```python
from build123d import *

# Parameters (mm, degrees)
SKETCH1_R           = 16.5
BOSS_EXTRUDE1_DEPTH = 6.5
BOSS_EXTRUDE1_TAPER = 6
SKETCH2_R           = 14.25
CUT_EXTRUDE1_DEPTH  = 4.5
CUT_EXTRUDE2_START  = -6
CUT_EXTRUDE2_DEPTH  = 6
CHAMFER1_SIZE       = 1.5


with BuildPart() as part:
    # Sketch1 → Boss-Extrude1 (new body)
    with BuildSketch(Plane(origin=(0, 0, 0), x_dir=(1, 0, 0), z_dir=(0, 1, 0))):
        Circle(SKETCH1_R)
    extrude(amount=BOSS_EXTRUDE1_DEPTH, taper=BOSS_EXTRUDE1_TAPER)

    # Sketch2 → Cut-Extrude1 (cut)
    with BuildSketch(Plane.XZ):
        with Locations(Location((0, 0, 0), (0, 0, 270))):
            Circle(SKETCH2_R)
    extrude(amount=-CUT_EXTRUDE1_DEPTH, mode=Mode.SUBTRACT)

    # Sketch3 → Cut-Extrude2 (cut)
    with BuildSketch(Plane(origin=(0, 6.5, 0), x_dir=(1, 0, 0), z_dir=(0, 1, 0)).offset(CUT_EXTRUDE2_START)):
        with BuildLine():
            Line((0, -14.25), (0, 14.25))
            ThreePointArc((0, 14.25), (14.25, 0), (0, -14.25))
        make_face()
    extrude(amount=CUT_EXTRUDE2_DEPTH, mode=Mode.SUBTRACT)

    # Chamfer1
    # the kernel refuses this chamfer: 1.5 mm, written as the material it takes off along each edge
    with BuildSketch(Plane(origin=(0, 4.5, 18.107524482), x_dir=(0.027495876610586376, 0.9996219169112968, 0), z_dir=(0, 0, -1))) as chamfer1_piece_1_section:
        Polygon((CHAMFER1_SIZE * 0.999621916911, -CHAMFER1_SIZE * 0.0274958766106), (-CHAMFER1_SIZE * 0.0274958766106, -CHAMFER1_SIZE * 0.999621916911), (0, 0), align=None)
    chamfer1_piece_1 = extrude(amount=36.215048964, mode=Mode.PRIVATE)
    chamfer1_piece_1 = chamfer1_piece_1 & Plane(origin=(0, 5.000185137, 0), x_dir=(0, 0, -1), z_dir=(0, -1, 0)) * Cylinder(14.25, 79, mode=Mode.PRIVATE)
    add(chamfer1_piece_1, mode=Mode.SUBTRACT)


solid = part.part
```
Here's how the part is built. I have some questions about the finished solid (model axes, mm). A direction names the side the tool comes from. Give positions to 0.01 mm unless a question says otherwise; leave off trailing zeros. Write each loop counter-clockwise with the first axis right and the second up, starting at its lowest first coordinate (ties: lowest second). Pieces come first, ordered by that corner, then holes.
(1) Thinking about a two-plate mould opening in X: for faces 1 (the face through (-1, 5, 0)), 2 (the face through (-3.47, 4.74, 15.62)), 3 (the face through (-6, 4.5, 0)), 4 (the face through (-4, 6.5, 0)), which applies, pulls with the +X half, pulls with the -X half, needs draft (parallel to the pull), parting line crosses it, or undercut?
Output values:
face 1: undercut
face 2: parting line crosses it
face 3: undercut
face 4: needs draft
(2) Will these pins go through, and if not, where does the flat tip stop? pin 1 (1.5 mm diameter, centred on x = -11, z = -1, fed in from -Y); pin 2 (2 mm diameter, centred on y = 5.5, z = 6, fed in from +X); pin 3 (12 mm diameter, centred on x = 5, z = 6.5, fed in from +Y); pin 4 (2 mm diameter, centred on y = 3.5, z = -12.5, fed in from +X).
Output values:
pin 1: stops at y = 4.5
pin 2: stops at x = 15.13
pin 3: stops at y = 6.5
pin 4: stops at x = 11.32
(3) On a 3-axis mill with a long thin cutter (end or side, diameter ignored), from which of +Z, -Z, +X, -X, +Y, -Y can I reach the whole of each face in a straight line? I mean faces 5 (the face through (-14, 0, 5)), 6 (the face through (14.13, 2.48, 1.86)). Say none if no direction works.
Output values:
face 5: +Z, -Z, +X, -X, -Y
face 6: -Y
(4) Imagine slicing it at A-A, the plane y = 1.5. Write out the boundary of the cut face in (x, z), and give its area (3 significant figures).
Output values:
outline: circle Ø32.68 at (0, 0); hole circle Ø28.5 at (0, 0)
area: 201 mm2
(5) If I drill on L1, parallel to Y at x = -5, z = -2; L2, parallel to X at y = 1.75, z = 1; L3, parallel to X at y = 2.25, z = -3, over which ranges is the centre line in solid material (lowest first)?
Output values:
L1: y = 4.5 to 6.5
L2: x = -16.29 to -14.21, 14.21 to 16.29
L3: x = -15.98 to -13.93, 13.93 to 15.98
